Here's how the part is built. I have some questions about the finished solid (model axes, mm). Face numbers are marked on the shaded views. A direction names the side the tool comes from. Round coordinates to 2 decimals unless told otherwise and drop trailing zeros. Write each loop counter-clockwise with the first axis right and the second up, starting at its lowest first coordinate (ties: lowest second). Pieces come first, ordered by that corner, then holes. Notation, with made-up numbers: (41, 65) -> (82, 65) arc R24 ccw to (82, 99) -> close; hole circle Ø4 at (5.25, 53.25). An arc over 180 degrees is marked (long way). Answer in a Markdown table with one row per item. Add a question column.
from build123d import *

# Parameters (mm, degrees)
SKETCH_R        = 6
PAD_DEPTH       = 22
POCKET_DEPTH    = 25
POCKET001_DEPTH = 8


with BuildPart() as part:
    # Sketch → Pad (new body)
    with BuildSketch(Plane.XY):
        Circle(SKETCH_R)
    extrude(amount=PAD_DEPTH)

    # Sketch003 → Pocket (cut)
    with BuildSketch(Plane(origin=(0, 0, 0), x_dir=(1, 0, 0), z_dir=(0, 0, -1))):
        with BuildLine():
            ThreePointArc((1.7, 0), (0, 1.7), (-1.7, 0))
            Line((-1.7, 0), (1.7, 0))
        make_face()
    extrude(amount=-POCKET_DEPTH, mode=Mode.SUBTRACT)

    # Sketch004 (on Face2 of Pocket) → Pocket001 (cut)
    with BuildSketch(Plane(origin=(0, 0, 0), x_dir=(1, 0, 0), z_dir=(0, 0, -1))):
        Polygon((4.4, 0), (2.2, 3.810512), (-2.2, 3.810512), (-4.4, 0), (-2.2, -3.810512), (2.2, -3.810512), align=None)
    extrude(amount=-POCKET001_DEPTH, mode=Mode.SUBTRACT)


solid = part.part
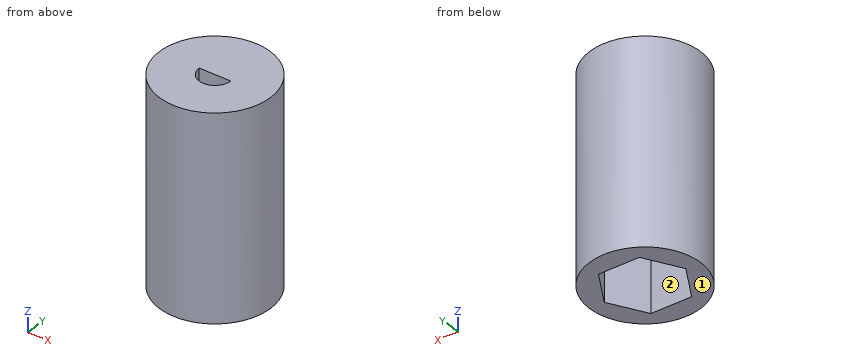
Item 1: If we section it at C-C on z = 15: Please give me the cut outline in (x, y).
Item 2: If we section it at D-D on x = 3.5: Please give me the cut outline in (y, z), then the cut area to 3 significant figures.
Item 3: For P1, Ø6, axis at y = 3.5, z = 2.5, coming from the +X side; P2, Ø1.3, axis at x = -1, z = 3, coming from the -Y side; P3, Ø2, axis at x = -4, z = 15, coming from the +Y side, each with a flat end and sliding along its axis, tell me the tip position at first contact or that it passes through.
Item 4: On a 3-axis mill with a long thin cutter (end or side, diameter ignored), from which of +Z, -Z, +X, -X, +Y, -Y can I reach the whole of each face in a straight line? I mean the marked faces 1 and 2. Say none if no direction works.
Item 5: If we section it at B-B on y = -0.25: Please give me the cut outline in (x, z), then the cut area to 3 significant figures.
Item 6: If we section it at A-A on x = 0: Please give me the cut outline in (y, z), then the cut area to 3 significant figures.
Item 7: I need wall thicknesses on line 1 along Y through (x, z) = (0, 3.5); line 2 along Z through (x, y) = (1, -1.75); line 3 along Y through (x, z) = (-1.25, 6). Which ranges of each line are inside material? Lowest first, please. Write a range as from..to.
Results list:
| question | item | result |
|---|---|---|
| 1 | outline | circle Ø12 at (0, 0); hole (-1.7, 0) arc R1.7 ccw to (1.7, 0) -> close |
| 2 | outline | (-4.87, 0) -> (-1.56, 0) -> (-1.56, 8) -> (1.56, 8) -> (1.56, 0) -> (4.87, 0) -> (4.87, 22) -> (-4.87, 22) -> close |
| 2 | area | 189 mm² |
| 3 | P1 | x = 5.98 |
| 3 | P2 | y = -5.99 |
| 3 | P3 | y = 5.2 |
| 4 | face 1 | -Z, +X, -X, +Y, -Y |
| 4 | face 2 | -Z |
| 5 | outline | (-5.99, 0) -> (-4.26, 0) -> (-4.26, 8) -> (-1.68, 8) -> (-1.68, 22) -> (-5.99, 22) -> close; (1.68, 8) -> (4.26, 8) -> (4.26, 0) -> (5.99, 0) -> (5.99, 22) -> (1.68, 22) -> close |
| 5 | area | 149 mm² |
| 6 | outline | (-6, 0) -> (-3.81, 0) -> (-3.81, 8) -> (-1.7, 8) -> (-1.7, 22) -> (-6, 22) -> close; (0, 8) -> (3.81, 8) -> (3.81, 0) -> (6, 0) -> (6, 22) -> (0, 22) -> close |
| 6 | area | 179 mm² |
| 7 | line 1 | -6..-3.81, 3.81..6 |
| 7 | line 2 | 8..22 |
| 7 | line 3 | -5.87..-3.81, 3.81..5.87 |
